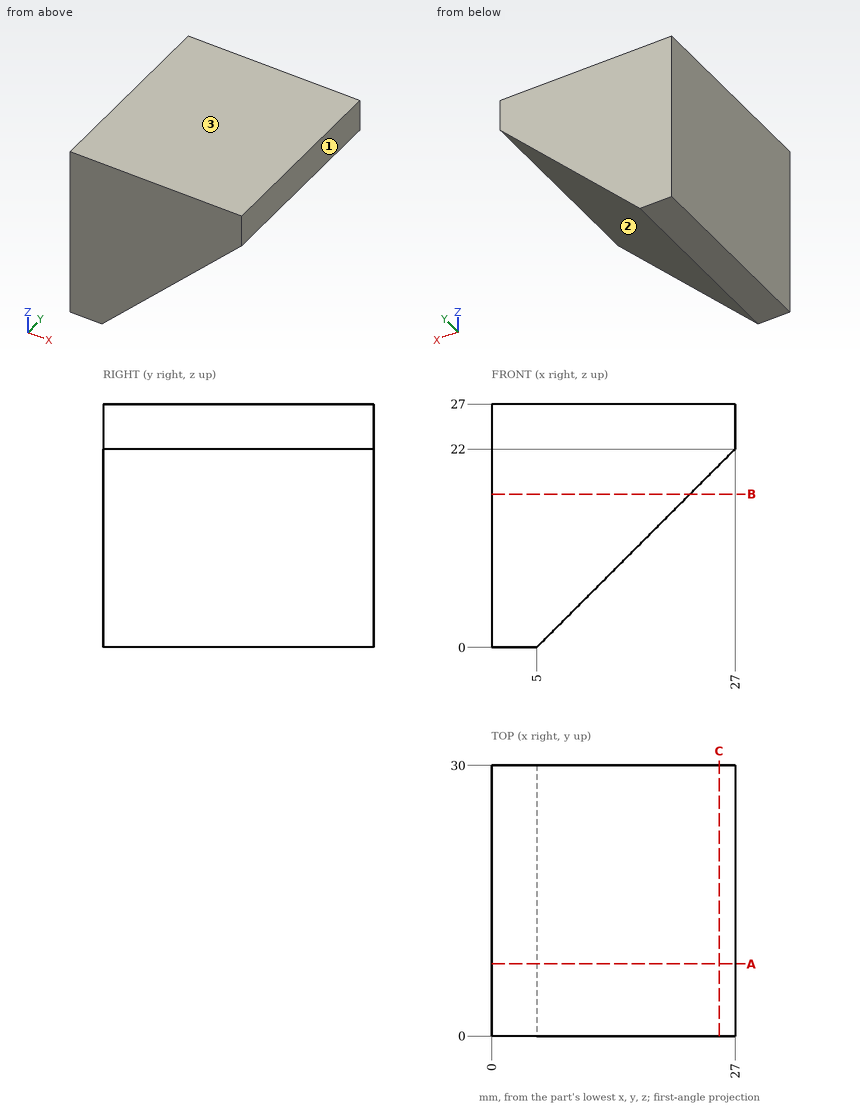
Answer from the drawing. Dimensions are ordinates in mm from the lowest x, y and z of the part. Round coordinates to 2 decimals unless told otherwise and drop trailing zeros. Write each loop counter-clockwise with the first axis right and the second up, starting at its lowest first coordinate (ties: lowest second). Pieces come first, ordered by that corner, then holes. Notation, with made-up numbers: M -12,-12.75 L 42,-12.75 A20 ccw 42,4.25 Z; hole C 80,-11.5 d10. An arc over 180 degrees is marked long. One line per item, written item: value.
Q1. Find section A-A on y = 8. Write down the section's boundary in (x, z).
Data:
outline: M 0,0 L 5,0 L 27,22 L 27,27 L 0,27 Z
Q2. Straight lines are drawn through the part: line 1 (Z direction, x = 15, y = 28.75); line 2 (X direction, y = 27, z = 10.25); line 3 (Z direction, x = 8.25, y = 8.5). For each, find the intervals that lie inside material, in ascending order. Write a range as [from, to].
Data:
line 1: [10, 27]
line 2: [0, 15.25]
line 3: [3.25, 27]
Q3. Flat-ended cylindrical pins translate along their axes: pin 1 Ø2 at (y, z) = (4, 9.5) entering from +X; pin 2 Ø6 at (x, y) = (14.5, 8) entering from -Z; pin 3 Ø10 at (y, z) = (16.5, 13.5) entering from +X. Find the tip coordinate at first contact, or state that the pin passes through.
Data:
pin 1: x = 15.5
pin 2: z = 6.5
pin 3: x = 23.5
Q4. Find section C-C on x = 25.25. Write down the section's boundary in (y, z).
Data:
outline: M 0,20.25 L 30,20.25 L 30,27 L 0,27 Z
Q5. Find section B-B on z = 17. Write down the section's boundary in (x, y), plus the area to 3 significant figures.
Data:
outline: M 0,0 L 22,0 L 22,30 L 0,30 Z
area: 660 mm2
Q6. For a pull along Z with two mould halves and no side action, classify the marked faces 1, 2 and 3 as +Z half, -Z half, draft (parallel to the pull), parting line (faces both ways), or undercut.
Data:
face 1: draft
face 2: -Z half
face 3: +Z half
